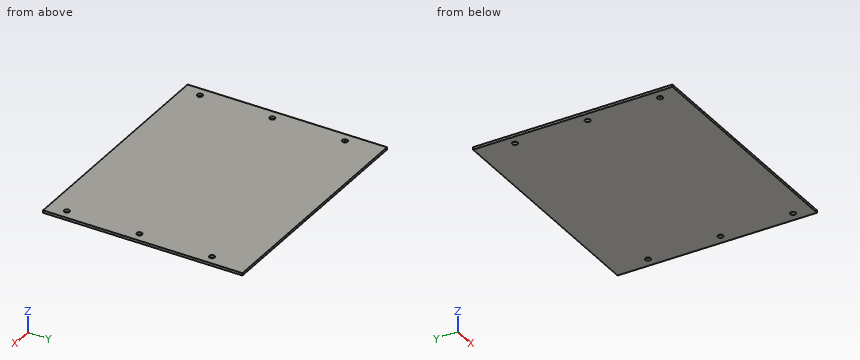
```python
from build123d import *

# Parameters (mm, degrees)
SKETCH_1_W          = 199
SKETCH_1_H          = 165
EXTRUDE_1_DEPTH     = 2
SKETCH_2_R          = 2.2
CUT_EXTRUDE_1_DEPTH = 2
SKETCH_3_R          = 2.2
CUT_EXTRUDE_2_DEPTH = 2


with BuildPart() as part:
    # ｽｹｯﾁ1 → ﾎﾞｽ - 押し出し1 (new body)
    with BuildSketch(Plane.XY):
        Rectangle(SKETCH_1_W, SKETCH_1_H)
    extrude(amount=EXTRUDE_1_DEPTH)

    # ｽｹｯﾁ2 → ｶｯﾄ - 押し出し1 (cut)
    with BuildSketch(Plane.XY.offset(2)):
        with Locations((-91.5, -67.5)):
            Circle(SKETCH_2_R)
        with Locations((-91.5, -7.5)):
            Circle(SKETCH_2_R)
        with Locations((-91.5, 52.5)):
            Circle(SKETCH_2_R)
    extrude(amount=-CUT_EXTRUDE_1_DEPTH, mode=Mode.SUBTRACT)

    # ｽｹｯﾁ3 → ｶｯﾄ - 押し出し2 (cut)
    with BuildSketch(Plane.XY.offset(2)):
        with Locations((91.5, -67.5)):
            Circle(SKETCH_3_R)
        with Locations((91.5, -7.5)):
            Circle(SKETCH_3_R)
        with Locations((91.5, 52.5)):
            Circle(SKETCH_3_R)
    extrude(amount=-CUT_EXTRUDE_2_DEPTH, mode=Mode.SUBTRACT)


solid = part.part
```
Can you work these out from the model? Positions are in its coordinate system, mm. Give positions to 0.01 mm unless a question says otherwise; leave off trailing zeros. Write each loop counter-clockwise with the first axis right and the second up, starting at its lowest first coordinate (ties: lowest second). Pieces come first, ordered by that corner, then holes. Notation, with made-up numbers: (8.5, 53.5) -> (36.5, 53.5) arc R24 cw to (36.5, 71.5) -> close; hole circle Ø8 at (-39.5, 26.5). An arc over 180 degrees is marked (long way). One line per item, written item: value.
Q1. Imagine slicing it at A-A on x = 91.5. Please give me the cut outline in (y, z).
Results found:
outline: (-82.5, 0) -> (-69.7, 0) -> (-69.7, 2) -> (-82.5, 2) -> close; (-65.3, 0) -> (-9.7, 0) -> (-9.7, 2) -> (-65.3, 2) -> close; (-5.3, 0) -> (50.3, 0) -> (50.3, 2) -> (-5.3, 2) -> close; (54.7, 0) -> (82.5, 0) -> (82.5, 2) -> (54.7, 2) -> close
Q2. Please list where these lines run through material, in increasing order: line 1 (Y direction, x = 91.5, z = 1.4); line 2 (X direction, y = -8.5, z = 0.85). Write a range as [from, to].
Results found:
line 1: y = [-82.5, -69.7], [-65.3, -9.7], [-5.3, 50.3], [54.7, 82.5]
line 2: x = [-99.5, -93.46], [-89.54, 89.54], [93.46, 99.5]
Q3. For P1, Ø5, axis at x = 91.5, y = -67.5, coming from the +Z side, with a flat end and sliding along its axis, tell me the tip position at first contact or that it passes through.
Results found:
P1: stops at z = 2
Q4. Imagine slicing it at B-B on y = 52.5. Please give me the cut outline in (x, z), and give its area (3 significant figures).
Results found:
outline: (-99.5, 0) -> (-93.7, 0) -> (-93.7, 2) -> (-99.5, 2) -> close; (-89.3, 0) -> (89.3, 0) -> (89.3, 2) -> (-89.3, 2) -> close; (93.7, 0) -> (99.5, 0) -> (99.5, 2) -> (93.7, 2) -> close
area: 380 mm^2
